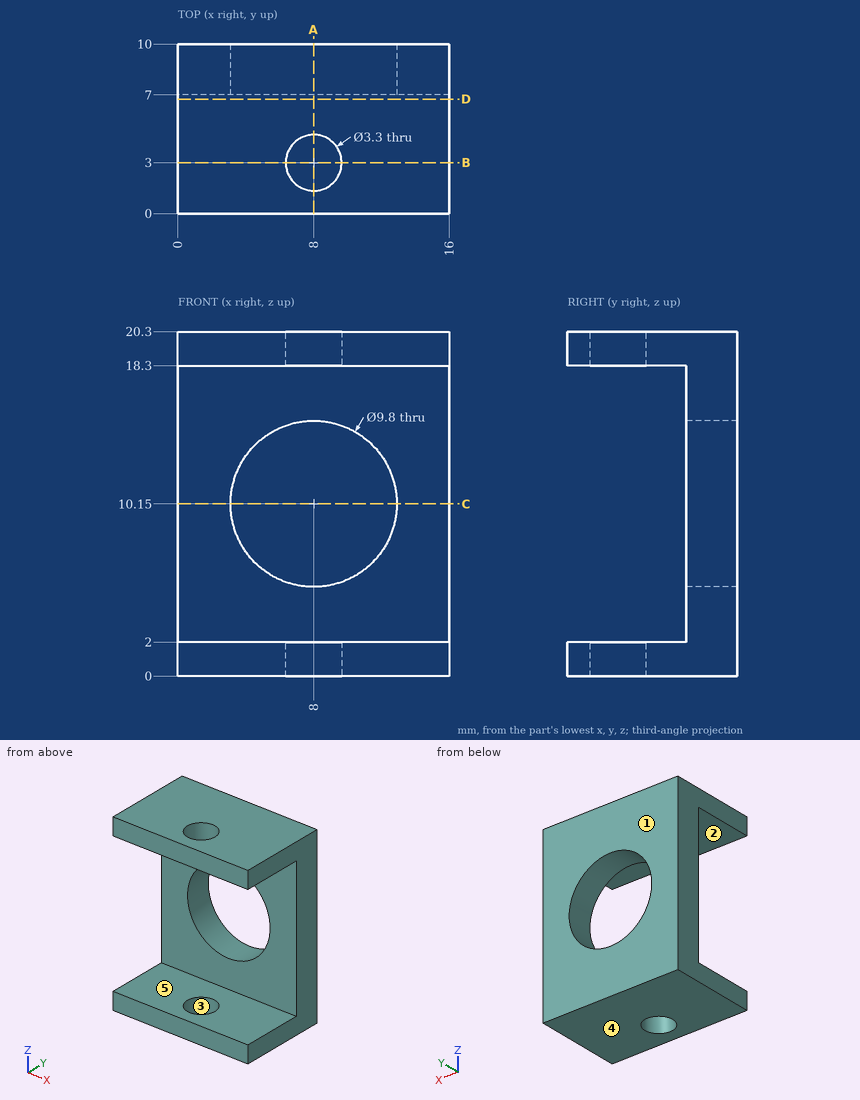
Source: three-view drawing plus pictorial views. Frame: mm from the lowest corner of the part. A direction names the side the tool comes from. Give positions to 0.01 mm unless a question says otherwise; leave off trailing zeros. Write each loop counter-clockwise with the first axis right and the second up, starting at its lowest first coordinate (ties: lowest second). Pieces come first, ordered by that corner, then holes. Notation, with made-up numbers: (20, 62.5) - (52, 62.5) arc R22 ccw to (52, 87.5) - close; hole circle Ø7 at (69.5, 20.5). An arc over 180 degrees is marked (long way). Write item = value, one per line. Start each with the question number.
1. Mould query, pull axis Z, two halves, no side actions, for the marked faces 3, 4 and 5. Classes: released by +Z, released by -Z, zero draft, split by the parting line, or undercut.
2. First-contact query: pin 1 Ø5 at (x, z) = (4.5, 12) entering from -Y; pin 2 Ø3 at (x, y) = (8, 3) entering from +Z; pin 3 Ø3.5 at (x, y) = (6, 3.5) entering from -Z. Flat tips, straight axial feed; report the tip coordinate or a pass-through.
3. Section query A-A, the plane x = 8. Output: boundary loops of the cut face in (y, z).
4. Section query C-C, the plane z = 10.15. Output: boundary loops of the cut face in (x, y), then the cut area to 3 significant figures.
5. Access query for the marked faces 1 and 2. Directions: +Z, -Z, +X, -X, +Y, -Y. A direction counts if a zero-diameter tool reaches every point of the face in a straight line with its end or side. Return the directions, or none.
6. Ray query, L1, parallel to Z at x = 13, y = 2.75; L2, parallel to Y at x = 8, z = 1.15; L3, parallel to Z at x = 7.75, y = 7.5. Return the intervals inside material, ascending.
7. Section query B-B, the plane y = 3. Output: boundary loops of the cut face in (x, z), then the cut area to 3 significant figures.
8. Section query D-D, the plane y = 6.75. Output: boundary loops of the cut face in (x, z), then the cut area to 3 significant figures.
Check sheet entries:
q1.face_3 = zero draft
q1.face_4 = released by -Z
q1.face_5 = undercut
q2.pin_1 = 7
q2.pin_2 = through
q2.pin_3 = 0
q3.outline = (0, 0) - (1.35, 0) - (1.35, 2) - (0, 2) - close; (0, 18.3) - (1.35, 18.3) - (1.35, 20.3) - (0, 20.3) - close; (4.65, 0) - (10, 0) - (10, 5.25) - (7, 5.25) - (7, 2) - (4.65, 2) - close; (4.65, 18.3) - (7, 18.3) - (7, 15.05) - (10, 15.05) - (10, 20.3) - (4.65, 20.3) - close
q4.outline = (0, 7) - (3.1, 7) - (3.1, 10) - (0, 10) - close; (12.9, 7) - (16, 7) - (16, 10) - (12.9, 10) - close
q4.area = 18.6 mm2
q5.face_1 = +Z, -Z, +X, -X, +Y
q5.face_2 = +X, -X, -Y
q6.L1 = 0 to 2, 18.3 to 20.3
q6.L2 = 0 to 1.35, 4.65 to 10
q6.L3 = 0 to 5.26, 15.04 to 20.3
q7.outline = (0, 0) - (6.35, 0) - (6.35, 2) - (0, 2) - close; (0, 18.3) - (6.35, 18.3) - (6.35, 20.3) - (0, 20.3) - close; (9.65, 0) - (16, 0) - (16, 2) - (9.65, 2) - close; (9.65, 18.3) - (16, 18.3) - (16, 20.3) - (9.65, 20.3) - close
q7.area = 50.8 mm2
q8.outline = (0, 0) - (16, 0) - (16, 2) - (0, 2) - close; (0, 18.3) - (16, 18.3) - (16, 20.3) - (0, 20.3) - close
q8.area = 64.0 mm2
